Geometry: final body of the model. Coordinates: model frame, mm. A direction names the side the tool comes from. Give positions to 0.01 mm unless a question says otherwise; leave off trailing zeros. Order: outer loops, then holes, each group sorted by start corner. A loop starts at its lowest first (then second) coordinate and runs counter-clockwise, first axis right, second up. Notation, with made-up numbers: M -18,83.5 L -11,83.5 A29 cw -11,113.5 Z; hole C 36,88 d5. An arc over 180 degrees is marked long. Use CSV: the item, a comma, the result in double quotes.
```python
from build123d import *

# Parameters (mm, degrees)
SKETCH_3_R         = 23
EXTRUDE_1_DEPTH    = 2
SKETCH_4_R         = 23
EXTRUDE_2_DEPTH    = 2
HOLE_WIZARD_M3_1_D = 3.4
SKETCH1_R          = 1
SKETCH1_R_2        = 3.25
CUT_EXTRUDE1_DEPTH = 37.249137921


with BuildPart() as part:
    # 草图2 → 旋转1 (revolve)
    with BuildSketch(Plane.XY):
        with BuildLine():
            Line((20, 6), (0, 6))
            Line((0, 6), (0, 0))
            Line((0, 0), (0, -6))
            Line((0, -6), (20, -6))
            add(Edge.make_bspline(
                [(20, 6), (10, 0), (20, -6)],
                knots=[0, 0, 0, 1, 1, 1], degree=2))
        make_face()
    revolve(axis=Axis((0, 6, 0), (0, -1, 0)))

    # 草图3 → 凸台-拉伸1 (add)
    with BuildSketch(Plane(origin=(0, 6, 0), x_dir=(1, 0, 0), z_dir=(0, 1, 0))):
        with Locations(Location((0, 0, 0), (0, 0, 270))):
            Circle(SKETCH_3_R)
    extrude(amount=EXTRUDE_1_DEPTH)

    # 草图4 → 凸台-拉伸2 (add)
    with BuildSketch(Plane.XZ.offset(6)):
        with Locations(Location((0, 0, 0), (0, 0, 90))):
            Circle(SKETCH_4_R)
    extrude(amount=EXTRUDE_2_DEPTH)

    # M3 间隙孔1 (through all)
    with Locations(Plane(origin=(0, 8, 0), x_dir=(1, 0, 0), z_dir=(0, 1, 0))):
        with Locations((0, -7), (0, 7), (-7, 0), (7, 0)):
            Hole(HOLE_WIZARD_M3_1_D / 2)

    # Sketch1 → Cut-Extrude1 (cut, through all)
    with BuildSketch(Plane(origin=(0, 8, 0), x_dir=(1, 0, 0), z_dir=(0, 1, 0))):
        with Locations(Location((0, 16, 0), (0, 0, 270))):
            Circle(SKETCH1_R)
        with Locations(Location((0, 0, 0), (0, 0, 270))):
            Circle(SKETCH1_R_2)
        with Locations(Location((4.938587697, 15.21875, 0), (0, 0, 270))):
            Circle(SKETCH1_R)
    extrude(amount=-CUT_EXTRUDE1_DEPTH, mode=Mode.SUBTRACT)


solid = part.part
```
1. Section A-A, the plane z = 0. Give the number of separate pieces and of enclosed holes in the cut face, plus the area to 3 significant figures.
Answer:
separate pieces,"4"
enclosed holes,"0"
area,"371 mm2"
2. Line query: line 1 (Y direction, x = -20.5, z = -2.5); line 2 (Z direction, x = -0.5, y = 5); line 3 (X direction, y = -3.75, z = 7). Output: solid intervals per line, ascending.
Answer:
line 1,"-8 to -6, 6 to 8"
line 2,"-18.47 to -16.87, -15.13 to -8.62, -5.38 to -3.21, 3.21 to 5.38, 8.62 to 18.47"
line 3,"-15.44 to -1.7, 1.7 to 15.44"
3. Pull-direction query (Z, two-part tool) for faces 3 (the face through (4.556, -4.831, -14.295)), 4 (the face through (0, -8, 5)), 5 (the face through (-19.394, -6.986, 12.365)); classes: +Z half, -Z half, draft (parallel to the pull), parting line (faces both ways), or undercut.
Answer:
face 3,"undercut"
face 4,"draft"
face 5,"parting line"
4. Pin query (flat end, axial travel): pin 1 Ø5 at (y, z) = (-1.5, -14.5) entering from -X; pin 2 Ø2 at (y, z) = (-2.5, -10.5) entering from -X; pin 3 Ø5 at (y, z) = (1, 0.5) entering from +X. Return the tip coordinate at first contact, or that it passes through.
Answer:
pin 1,"x = -10.49"
pin 2,"x = -13.22"
pin 3,"x = 16.69"
5. Reachability of faces 1 (the face through (19, 6, -7)), 2 (the face through (19.394, 6.986, 12.365)) from +Z, -Z, +X, -X, +Y, -Y: full face, straight path, thin tool, end or side. Return the list, or none.
Answer:
face 1,"none"
face 2,"+Y, -Y"
6. Section B-B, the plane y = 6.75. Return the cut outline in (x, z).
Answer:
outline,"C 0,0 d46; hole C -7,0 d3.4; hole C 0,0 d6.5; hole C 0,-7 d3.4; hole C 0,7 d3.4; hole C 0,-16 d2; hole C 4.94,-15.22 d2; hole C 7,0 d3.4"
